Build history of the part. All positions in model axes, mm. Face numbers are marked on the shaded views. A direction names the side the tool comes from. Coordinates: 2 decimals unless noted, no trailing zeros. Order: outer loops, then holes, each group sorted by start corner. A loop starts at its lowest first (then second) coordinate and runs counter-clockwise, first axis right, second up. Notation, with made-up numbers: (10.5, 11.25) - (40.5, 11.25) arc R15 ccw to (40.5, 24.25) - close; hole circle Ø2 at (56, 63.5). An arc over 180 degrees is marked (long way). Write each question's results on one line, items separated by ' | '. Start each with the question number.
from build123d import *

# Parameters (mm, degrees)
F0_W      = 90.424
F0_H      = 144.78
F1_DEPTH  = 40.005
F2_W      = 155.254013
F2_H      = 39.959349
F2_W_2    = 138.807609
F2_H_2    = 17.542356
F3_DEPTH  = 30.226
F4_R      = 1.524
F5_R      = 2.2225
F6_DEPTH  = 25.4
F7_W      = 25.824266
F7_H      = 100.72116
F8_DEPTH  = 27.94
F9_W      = 7.62
F9_H      = 11.43
F10_DEPTH = 12.7
F11_R     = 1.524
F12_W     = 6.096
F12_H     = 7.62
F12_H_2   = 10.16
F13_DEPTH = 10.16


with BuildPart() as f1:
    # F0 (on Top) → F1 (new body)
    with BuildSketch(Plane.XY):
        Rectangle(F0_W, F0_H)
    extrude(amount=F1_DEPTH)

    # F2 (on face) → F3 (cut)
    with BuildSketch(Plane.XY.offset(40.005)):
        with Locations((-0.908692, -82.463674)):
            Rectangle(F2_W, F2_H)
        with Locations((-0.57976, 71.255178)):
            Rectangle(F2_W_2, F2_H_2)
    extrude(amount=-F3_DEPTH, mode=Mode.SUBTRACT)

    # F4
    f4_edges = [f1.edges().sort_by_distance(p)[0] for p in [
        (45.212, -72.39, 4.8895),
        (-45.212, -72.39, 4.8895),
        (45.212, 72.39, 4.8895),
        (-45.212, 72.39, 4.8895),
    ]]
    fillet(f4_edges, radius=F4_R)

    # F5 (on face) → F6 (cut)
    with BuildSketch(Plane(origin=(0, 0, 0), x_dir=(1, 0, 0), z_dir=(0, 0, -1))):
        with Locations((-34.925, 67.31)):
            Circle(F5_R)
        with Locations((34.925, 67.31)):
            Circle(F5_R)
        with Locations((34.925, -67.31)):
            Circle(F5_R)
        with Locations((-34.925, -67.31)):
            Circle(F5_R)
    extrude(amount=-F6_DEPTH, mode=Mode.SUBTRACT)

    # F7 (on face) → F8 (cut)
    with BuildSketch(Plane.XY.offset(40.005)):
        with Locations((-48.345133, 0)):
            Rectangle(F7_W, F7_H)
        with Locations((48.345133, 0)):
            Rectangle(F7_W, F7_H)
    extrude(amount=-F8_DEPTH, mode=Mode.SUBTRACT)

    # F9 (on face) → F10 (join)
    with BuildSketch(Plane.XY.offset(12.065)):
        with Locations((39.243, 39.56558)):
            Rectangle(F9_W, F9_H)
        with Locations((39.243, 23.61438)):
            Rectangle(F9_W, F9_H)
        with Locations((39.243, -23.83282)):
            Rectangle(F9_W, F9_H)
        with Locations((39.243, -39.78402)):
            Rectangle(F9_W, F9_H)
    extrude(amount=F10_DEPTH)

    # F11
    f11_edges = [f1.edges().sort_by_distance(p)[0] for p in [
        (39.243, -45.49902, 24.765),
        (39.243, -34.06902, 24.765),
        (39.243, -29.54782, 24.765),
        (39.243, -18.11782, 24.765),
        (39.243, 17.89938, 24.765),
        (39.243, 33.85058, 24.765),
        (39.243, 29.32938, 24.765),
        (39.243, 45.28058, 24.765),
    ]]
    fillet(f11_edges, radius=F11_R)

    # F12 (on face) → F13 (join)
    with BuildSketch(Plane.XY.offset(12.065)):
        with Locations((-39.243, -34.35858)):
            Rectangle(F12_W, F12_H)
        with Locations((-39.243, -9.89838)):
            Rectangle(F12_W, F12_H_2)
    extrude(amount=F13_DEPTH)


solid = f1.part
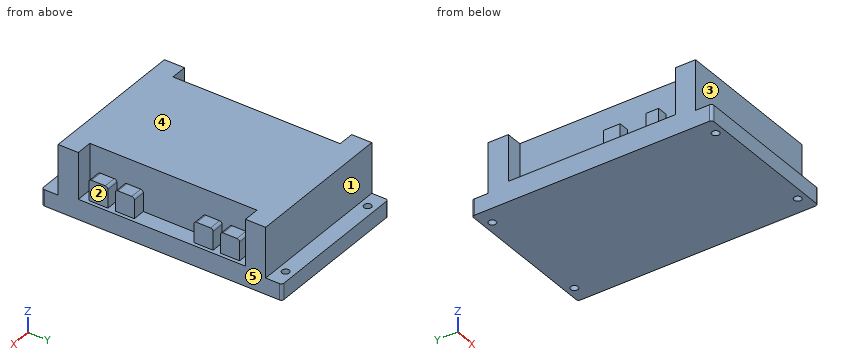
Item 1: Slice it at A-A (y = 67.31). Write the cut outline in (x, z), then the cut area to 3 significant figures.
Item 2: Which spindle directions (+Z, -Z, +X, -X, +Y, -Y) get a long thin tool onto all of the face, cutting with end or side? Do the marked faces 1, 2, 3, 4 and 5. Say none if no direction does.
Item 3: Slice it at D-D (x = -5.5). Write the cut outline in (y, z) (3 decimals).
Item 4: Slice it at B-B (z = 28). Write the cut outline in (x, y).
Item 5: Probe probe 1 along X at (y, z) = (67.31, 4); probe 2 along Y at (x, z) = (38.5, 22.5); probe 3 along Y at (x, z) = (-5, 10.5). List the from-to ranges inside material, lowest first.
Item 6: Flat gauge pins, fed straight in: P1, Ø1.8, axis at x = -38, z = 17, coming from the -Y side; P2, Ø2, axis at x = -2, z = 24.5, coming from the +Y side; P3, Ø8, axis at y = -8.5, z = 17, coming from the -X side. Where does each tip first touch, or does it go through?
Item 7: Slice it at C-C (y = 41). Write the cut outline in (x, z) (3 decimals), then the cut area to 3 significant figures.
Resolved:
1) outline: (-45.21, 0) - (-37.15, 0) - (-37.15, 9.78) - (-45.21, 9.78) - close; (-32.7, 0) - (32.7, 0) - (32.7, 9.78) - (-32.7, 9.78) - close; (37.15, 0) - (45.21, 0) - (45.21, 9.78) - (37.15, 9.78) - close | area: 797 mm^2
2) face 1: +Z, +X, -X, +Y | face 2: +Z, +X | face 3: +Z, +X, -X, -Y | face 4: +Z, +X, -X, +Y, -Y | face 5: +Z, -Z, +X, +Y, -Y
3) outline: (-72.39, 0) - (72.39, 0) - (72.39, 9.779) - (62.484, 9.779) - (62.484, 40.005) - (-62.484, 40.005) - (-62.484, 9.779) - (-72.39, 9.779) - close
4) outline: (-45.21, -62.48) - (45.21, -62.48) - (45.21, -50.36) - (35.43, -50.36) - (35.43, 50.36) - (45.21, 50.36) - (45.21, 62.48) - (-45.21, 62.48) - (-45.21, 50.36) - (-35.43, 50.36) - (-35.43, -50.36) - (-45.21, -50.36) - close
5) probe 1: -45.21 to -37.15, -32.7 to 32.7, 37.15 to 45.21 | probe 2: -62.48 to -50.36, -45.5 to -34.07, -29.55 to -18.12, 17.9 to 29.33, 33.85 to 45.28, 50.36 to 62.48 | probe 3: -62.48 to 62.48
6) P1: y = -62.48 | P2: y = 62.48 | P3: x = -42.29
7) outline: (-45.212, 0) - (45.212, 0) - (45.212, 12.065) - (43.053, 12.065) - (43.053, 24.765) - (35.433, 24.765) - (35.433, 40.005) - (-35.433, 40.005) - (-35.433, 12.065) - (-45.212, 12.065) - close | area: 3,170 mm^2
